```python
from build123d import *

# Parameters (mm, degrees)
SKETCH1_W           = 132
SKETCH1_H           = 160
BOSS_EXTRUDE1_DEPTH = 6
SKETCH3_W           = 32
SKETCH3_H           = 54
SKETCH3_W_2         = 26
SKETCH3_H_2         = 48
BOSS_EXTRUDE2_DEPTH = 17.5
SKETCH4_W           = 32
SKETCH4_H           = 54
BOSS_EXTRUDE3_DEPTH = 3
SKETCH5_W           = 25
SKETCH5_H           = 17
CUT_EXTRUDE1_DEPTH  = 3
SKETCH6_W           = 12
SKETCH6_H           = 54
BOSS_EXTRUDE4_DEPTH = 3
SKETCH7_R           = 1.6
CUT_EXTRUDE2_DEPTH  = 106.177231376
SKETCH8_W           = 3
SKETCH8_H           = 6.5
BOSS_EXTRUDE5_DEPTH = 20
SKETCH9_R           = 1.55
CUT_EXTRUDE3_DEPTH  = 6
SKETCH10_R          = 1.6
CUT_EXTRUDE4_DEPTH  = 108.043215572
SKETCH11_W          = 2.5
SKETCH11_H          = 7
BOSS_EXTRUDE6_DEPTH = 19.36
SKETCH12_R          = 1.6
CUT_EXTRUDE5_DEPTH  = 19.36
SKETCH13_W          = 3
SKETCH13_H          = 7
BOSS_EXTRUDE7_DEPTH = 15
SKETCH14_R          = 2
CUT_EXTRUDE6_DEPTH  = 15
CUT_EXTRUDE7_START  = -6
CUT_EXTRUDE7_DEPTH  = 6
SKETCH16_R          = 1.6
CUT_EXTRUDE8_DEPTH  = 15


# Read off the part's stored shape, not the designer's step: Cut-Extrude7
with BuildPart() as part:
    # Sketch1 → Boss-Extrude1 (new body)
    with BuildSketch(Plane.XY):
        Rectangle(SKETCH1_W, SKETCH1_H)
    extrude(amount=BOSS_EXTRUDE1_DEPTH)

    # Sketch3 → Boss-Extrude2 (add)
    with BuildSketch(Plane.XY.offset(6)):
        with Locations((0, -53)):
            Rectangle(SKETCH3_W, SKETCH3_H)
        with Locations((0, -53)):
            Rectangle(SKETCH3_W_2, SKETCH3_H_2, mode=Mode.SUBTRACT)
    extrude(amount=BOSS_EXTRUDE2_DEPTH)

    # Sketch4 → Boss-Extrude3 (add)
    with BuildSketch(Plane.XY.offset(23.5)):
        with Locations((0, -53)):
            Rectangle(SKETCH4_W, SKETCH4_H)
    extrude(amount=BOSS_EXTRUDE3_DEPTH)

    # Sketch5 → Cut-Extrude1 (cut)
    with BuildSketch(Plane.XZ.offset(80)):
        with Locations((0, 14.5)):
            Rectangle(SKETCH5_W, SKETCH5_H)
    extrude(amount=-CUT_EXTRUDE1_DEPTH, mode=Mode.SUBTRACT)

    # Sketch6 → Boss-Extrude4 (add)
    with BuildSketch(Plane.XY.offset(6)):
        with Locations((-22, -53)):
            Rectangle(SKETCH6_W, SKETCH6_H)
        with Locations((22, -53)):
            Rectangle(SKETCH6_W, SKETCH6_H)
    extrude(amount=BOSS_EXTRUDE4_DEPTH)

    # Sketch7 → Cut-Extrude2 (cut, through all)
    with BuildSketch(Plane.XY.offset(9)):
        with Locations((-22, -69)):
            Circle(SKETCH7_R)
        with Locations((-22, -33)):
            Circle(SKETCH7_R)
        with Locations(Location((22, -69, 0), (0, 0, 180))):
            Circle(SKETCH7_R)
        with Locations(Location((22, -33, 0), (0, 0, 180))):
            Circle(SKETCH7_R)
    extrude(amount=-CUT_EXTRUDE2_DEPTH, mode=Mode.SUBTRACT)

    # Sketch8 → Boss-Extrude5 (add)
    with BuildSketch(Plane.XY.offset(6)):
        with Locations((-54.38, -76.75)):
            Rectangle(SKETCH8_W, SKETCH8_H)
        with Locations((-54.38, -30.25)):
            Rectangle(SKETCH8_W, SKETCH8_H)
    boss_extrude5 = extrude(amount=BOSS_EXTRUDE5_DEPTH)

    # Sketch9 → Cut-Extrude3 (cut)
    with BuildSketch(Plane.ZY.offset(55.88)):
        with Locations((10.35, -76.75)):
            Circle(SKETCH9_R)
        with Locations((19.65, -76.75)):
            Circle(SKETCH9_R)
        with Locations((10.35, -30.25)):
            Circle(SKETCH9_R)
        with Locations((19.65, -30.25)):
            Circle(SKETCH9_R)
    cut_extrude3 = extrude(amount=-CUT_EXTRUDE3_DEPTH, mode=Mode.SUBTRACT)

    # Mirror1: Boss-Extrude5, Cut-Extrude3 across plane
    add(boss_extrude5.mirror(Plane(origin=(0, 0, 0), x_dir=(0, 0, 1), z_dir=(1, 0, 0))))
    add(cut_extrude3.mirror(Plane(origin=(0, 0, 0), x_dir=(0, 0, 1), z_dir=(1, 0, 0))), mode=Mode.SUBTRACT)

    # Sketch10 → Cut-Extrude4 (cut, through all)
    with BuildSketch(Plane(origin=(0, 0, 0), x_dir=(-1, 0, 0), z_dir=(0, 0, -1))):
        with Locations((-24.1, -75.572749788)):
            Circle(SKETCH10_R)
        with Locations((-21.15, -12.732749788)):
            Circle(SKETCH10_R)
        with Locations(Location((21.15, -12.732749788, 0), (0, 0, 180))):
            Circle(SKETCH10_R)
        with Locations((24.1, -75.572749788)):
            Circle(SKETCH10_R)
    extrude(amount=-CUT_EXTRUDE4_DEPTH, mode=Mode.SUBTRACT)

    # Sketch11 → Boss-Extrude6 (add)
    with BuildSketch(Plane(origin=(0, 0, 0), x_dir=(-1, 0, 0), z_dir=(0, 0, -1))):
        with Locations((-17.9, 1.267250212)):
            Rectangle(SKETCH11_W, SKETCH11_H)
        with Locations((-17.9, 50.267250212)):
            Rectangle(SKETCH11_W, SKETCH11_H)
    extrude(amount=BOSS_EXTRUDE6_DEPTH)

    # Sketch12 → Cut-Extrude5 (cut)
    with BuildSketch(Plane(origin=(19.15, 0, 0), x_dir=(0, 0, -1), z_dir=(1, 0, 0))):
        with Locations(Location((4.5, 50.267250212, 0), (0, 0, 90))):
            Circle(SKETCH12_R)
        with Locations(Location((14.5, 50.267250212, 0), (0, 0, 90))):
            Circle(SKETCH12_R)
        with Locations(Location((4.5, 1.267250212, 0), (0, 0, 90))):
            Circle(SKETCH12_R)
        with Locations(Location((14.5, 1.267250212, 0), (0, 0, 90))):
            Circle(SKETCH12_R)
    extrude(amount=-CUT_EXTRUDE5_DEPTH, mode=Mode.SUBTRACT)

    # Sketch13 → Boss-Extrude7 (add)
    with BuildSketch(Plane(origin=(0, 0, 0), x_dir=(-1, 0, 0), z_dir=(0, 0, -1))):
        with Locations((29.35, 35.967250212)):
            Rectangle(SKETCH13_W, SKETCH13_H)
    extrude(amount=BOSS_EXTRUDE7_DEPTH)

    # Sketch14 → Cut-Extrude6 (cut)
    with BuildSketch(Plane.ZY.offset(30.85)):
        with Locations((-9.9, 35.967250212)):
            Circle(SKETCH14_R)
    extrude(amount=-CUT_EXTRUDE6_DEPTH, mode=Mode.SUBTRACT)

    # Cut-Extrude7 outline → Cut-Extrude7 (cut)
    with BuildSketch(Plane(origin=(0, 0, 0), x_dir=(-1, 0, 0), z_dir=(0, 0, -1)).offset(CUT_EXTRUDE7_START)):
        Polygon((-30.85, 56.767250212), (30.85, 56.767250212), (30.85, -24), (58.88, -24), (58.88, -80), (66, -80), (66, 80), (-66, 80), (-66, -80), (-58.88, -80), (-58.88, -24), (-30.85, -24), align=None)
    extrude(amount=CUT_EXTRUDE7_DEPTH, mode=Mode.SUBTRACT)

    # Sketch16 → Cut-Extrude8 (cut)
    with BuildSketch(Plane(origin=(0, 0, 0), x_dir=(-1, 0, 0), z_dir=(0, 0, -1))):
        Circle(SKETCH16_R)
        with Locations((0, 52.767250212)):
            Circle(SKETCH16_R)
    extrude(amount=-CUT_EXTRUDE8_DEPTH, mode=Mode.SUBTRACT)


solid = part.part
```
Here's how the part is built. I have some questions about the finished solid (model axes, mm). A direction names the side the tool comes from. Give positions to 0.01 mm unless a question says otherwise; leave off trailing zeros. Write each loop counter-clockwise with the first axis right and the second up, starting at its lowest first coordinate (ties: lowest second). Pieces come first, ordered by that corner, then holes. Notation, with made-up numbers: M 14,59.25 L 25,59.25 A30 cw 25,88.25 Z; hole C -21,-18 d2. An arc over 180 degrees is marked long. Put each result on its own line as item: value. Start each with the question number.
Item 1: Thinking about a two-plate mould opening in Y: for faces 6 (the cylindrical face through (-29.37, 37.95, -10.16)), 7 (the flat face through (-14, -80, 10)), 8 (the flat face through (-12.5, -79, 14)), which applies, +Y half, -Y half, draft (parallel to the pull), parting line (faces both ways), or undercut?
Item 2: I need wall thicknesses on L1, parallel to X at y = -69, z = 3.5; L2, parallel to Z at x = 54, y = -30; L3, parallel to X at y = -62.5, z = 9.5. Which ranges of each line are inside material? Lowest first, please. Write a range as from..to.
Item 3: If we section it at B-B, the plane x = 0: Write out the boundary of the cut face in (y, z).
Item 4: Will these pins go through, and if not, where does the flat tip stop? pin 1 (3.5 mm diameter, centred on y = -76.75, z = 19.65, fed in from +X); pin 2 (1.5 mm diameter, centred on x = -55, y = -76.5, fed in from +Z); pin 3 (10 mm diameter, centred on x = -18, y = -10, fed in from +Z).
Item 5: On a 3-axis mill with a long thin cutter (end or side, diameter ignored), from which of +Z, -Z, +X, -X, +Y, -Y can I reach the whole of each face in a straight line? I mean faces 1 (the flat face through (54, -33.5, 16)), 2 (the cylindrical face through (54.401, -28.713, 10.148)), 3 (the flat face through (0, -26, 16)), 4 (the flat face through (-54, -30, 26)), 5 (the flat face through (54, -77, 26)). Say none if no direction works.
Item 6: If we section it at C-C, the plane x = -45: Write out the boundary of the cut face in (y, z), then the cut area to 3 significant figures.
Item 7: If we section it at A-A, the plane z = -4.5: Write out the boundary of the cut face in (x, y), then the cut area to 3 significant figures.
Values:
1. face 6: undercut
1. face 7: -Y half
1. face 8: draft
2. L1: -58.88..-23.6, -20.4..20.4, 23.6..58.88
2. L2: 0..8.82, 11.88..18.12, 21.18..26
2. L3: -16..-13, 13..16
3. outline: M -80,0 L -1.6,0 L -1.6,6 L -26,6 L -26,26.5 L -80,26.5 L -80,23 L -77,23 L -77,23.5 L -29,23.5 L -29,6 L -80,6 Z; M 1.6,0 L 51.17,0 L 51.17,6 L 1.6,6 Z; M 54.37,0 L 56.77,0 L 56.77,6 L 54.37,6 Z
4. pin 1: x = 55.88
4. pin 2: z = 26
4. pin 3: z = 6
5. face 1: +Z, +X
5. face 2: +X
5. face 3: +Z, +X, -X, +Y
5. face 4: +Z, -X, +Y, -Y
5. face 5: +Z, +X, +Y, -Y
6. outline: M -80,0 L -24,0 L -24,6 L -80,6 Z
6. area: 336 mm²
7. outline: M -30.85,32.47 L -27.85,32.47 L -27.85,39.47 L -30.85,39.47 Z; M 16.65,-2.23 L 19.15,-2.23 L 19.15,-0.33 L 16.65,-0.33 Z; M 16.65,2.87 L 19.15,2.87 L 19.15,4.77 L 16.65,4.77 Z; M 16.65,46.77 L 19.15,46.77 L 19.15,48.67 L 16.65,48.67 Z; M 16.65,51.87 L 19.15,51.87 L 19.15,53.77 L 16.65,53.77 Z
7. area: 40.0 mm²
